The model under review builds one solid part; all positions refer to its coordinate system, in mm. A direction names the side the tool comes from. Coordinates: 2 decimals unless noted, no trailing zeros. Write each loop counter-clockwise with the first axis right and the second up, starting at its lowest first coordinate (ties: lowest second). Pieces come first, ordered by that corner, then holes. Notation, with made-up numbers: (45.5, 72) - (77.5, 72) arc R27 cw to (77.5, 103) - close; hole circle Ø7 at (10.5, 5). An arc over 180 degrees is marked (long way). Return JSON: item names as keys, results as strings. Group by question number.
(1) Draft analysis for pull direction Y (two halves, no side actions). For faces 4 (the face through (-33.295, 2.242, -3.882)), 5 (the face through (-26.957, 22.715, -4.126)), 6 (the face through (-32.65, 5.08, -4.71)), state which applies: released by +Y, released by -Y, zero draft, split by the parting line, or undercut.
(2) We need section B-B on z = -3.81. State the section outline as (x, y) points (3 decimals), then the cut area to 3 significant figures.
(3) We need section D-D on y = 3.25. State the section outline as (x, z) points (3 decimals).
(4) We need section C-C on x = -12.7. State the section outline as (y, z) points.
(5) We need section A-A on y = 6.35. State the section outline as (x, z) points, then the cut area to 3 significant figures.
(6) For pin 1 Ø4 at (y, z) = (19, -4) entering from -X; pin 2 Ø2 at (y, z) = (12.5, -2.5) entering from +X; pin 3 Ø4 at (x, z) = (-34.925, -3.81) entering from +Y; pin 4 Ø2.5 at (x, y) = (-12.7, 6.35) entering from -Z, all flat-tipped, find the tip position at first contact; note any pin that passes through.
(7) To check wall thickness, follow L1, parallel to Y at x = -25.4, z = -3.5; L2, parallel to X at y = 6.35, z = -5.5; L3, parallel to Y at x = -13, z = -2.5. State the ranges of each line that lie inside material, in increasing order. Write a range as from..to.
(8) Tool access review of faces 1 (the face through (-7.62, 16, -4)), 2 (the face through (-30.48, 16, -4)), 3 (the face through (-14.208, 5.725, -4.126)): name each direction out of +Z, -Z, +X, -X, +Y, -Y from which nothing blocks a thin tool from reaching the whole face with its end or side.
```python
from build123d import *

# Parameters (mm, degrees)
SKETCH1_W                       = 38.1
SKETCH1_H                       = 7.62
BOSS_EXTRUDE1_DEPTH             = 5.08
SKETCH2_W                       = 22.86
SKETCH2_H                       = 7.62
BOSS_EXTRUDE2_DEPTH             = 22.86
F_4_CLEARANCE_HOLE1_D           = 3.2639
F_4_CLEARANCE_HOLE1_CSINK_D     = 4.5339
F_4_CLEARANCE_HOLE1_CSINK_ANGLE = 100
F_4_CLEARANCE_HOLE2_D           = 3.2639
F_4_CLEARANCE_HOLE2_CSINK_D     = 4.5339
F_4_CLEARANCE_HOLE2_CSINK_ANGLE = 100


with BuildPart() as part:
    # Sketch1 → Boss-Extrude1 (new body)
    with BuildSketch(Plane(origin=(0, 0, 0), x_dir=(1, 0, 0), z_dir=(0, 1, 0))):
        with Locations((-19.05, 3.81)):
            Rectangle(SKETCH1_W, SKETCH1_H)
    extrude(amount=BOSS_EXTRUDE1_DEPTH)

    # Sketch2 → Boss-Extrude2 (add)
    with BuildSketch(Plane(origin=(0, 5.08, 0), x_dir=(1, 0, 0), z_dir=(0, 1, 0))):
        with Locations((-19.05, 3.81)):
            Rectangle(SKETCH2_W, SKETCH2_H)
    extrude(amount=BOSS_EXTRUDE2_DEPTH)

    # #4 Clearance Hole1 (through all)
    with Locations(Plane(origin=(-25.4, 6.35, 0), x_dir=(1, 0, 0), z_dir=(0, 0, 1))):
        with Locations((0, 0), (0, 15.875), (12.7, 15.875), (12.7, 0)):
            CounterSinkHole(F_4_CLEARANCE_HOLE1_D / 2, F_4_CLEARANCE_HOLE1_CSINK_D / 2, counter_sink_angle=F_4_CLEARANCE_HOLE1_CSINK_ANGLE)

    # #4 Clearance Hole2 (through all)
    with Locations(Plane(origin=(0, 5.08, 0), x_dir=(1, 0, 0), z_dir=(0, 1, 0))):
        with Locations((-34.925, 3.81), (-3.175, 3.81)):
            CounterSinkHole(F_4_CLEARANCE_HOLE2_D / 2, F_4_CLEARANCE_HOLE2_CSINK_D / 2, counter_sink_angle=F_4_CLEARANCE_HOLE2_CSINK_ANGLE)


solid = part.part
```
Ans:
{
 "1": {"face 4": "zero draft", "face 5": "undercut", "face 6": "released by +Y"},
 "2": {"outline": "(-38.1, 0) - (-36.557, 0) - (-36.557, 4.547) - (-37.192, 5.08) - (-38.1, 5.08) - close; (-33.293, 0) - (-4.807, 0) - (-4.807, 4.547) - (-5.442, 5.08) - (-7.62, 5.08) - (-7.62, 27.94) - (-30.48, 27.94) - (-30.48, 5.08) - (-32.658, 5.08) - (-33.293, 4.547) - close; (-1.543, 0) - (0, 0) - (0, 5.08) - (-0.908, 5.08) - (-1.543, 4.547) - close; hole circle Ø3.264 at (-25.4, 6.35); hole circle Ø3.264 at (-25.4, 22.225); hole circle Ø3.264 at (-12.7, 6.35); hole circle Ø3.264 at (-12.7, 22.225)", "area": "649 mm²"},
 "3": {"outline": "(-38.1, -7.62) - (0, -7.62) - (0, 0) - (-38.1, 0) - close; hole circle Ø3.264 at (-34.925, -3.81); hole circle Ø3.264 at (-3.175, -3.81)"},
 "4": {"outline": "(0, -7.62) - (4.72, -7.62) - (4.72, -0.53) - (4.08, 0) - (0, 0) - close; (7.98, -7.62) - (20.59, -7.62) - (20.59, -0.53) - (19.96, 0) - (8.62, 0) - (7.98, -0.53) - close; (23.86, -7.62) - (27.94, -7.62) - (27.94, 0) - (24.49, 0) - (23.86, -0.53) - close"},
 "5": {"outline": "(-30.48, -7.62) - (-27.03, -7.62) - (-27.03, -0.53) - (-27.67, 0) - (-30.48, 0) - close; (-23.77, -7.62) - (-14.33, -7.62) - (-14.33, -0.53) - (-14.97, 0) - (-23.13, 0) - (-23.77, -0.53) - close; (-11.07, -7.62) - (-7.62, -7.62) - (-7.62, 0) - (-10.43, 0) - (-11.07, -0.53) - close", "area": "124 mm²"},
 "6": {"pin 1": "x = -30.48", "pin 2": "x = -7.62", "pin 3": "y = 4.86", "pin 4": "through"},
 "7": {"L1": "0..4.72, 7.98..20.59, 23.86..27.94", "L2": "-30.48..-27.03, -23.77..-14.33, -11.07..-7.62", "L3": "0..4.75, 7.95..20.62, 23.83..27.94"},
 "8": {"face 1": "+Z, -Z, +X, +Y", "face 2": "+Z, -Z, -X, +Y", "face 3": "+Z, -Z"}
}
